Geometry: final body of the model. Coordinates: model frame, mm. A direction names the side the tool comes from. Give positions to 0.01 mm unless a question says otherwise; leave off trailing zeros. Write each loop counter-clockwise with the first axis right and the second up, starting at its lowest first coordinate (ties: lowest second). Pieces come first, ordered by that corner, then holes.
Q1. Section A-A (x = 4). Return the cut outline in (y, z), plus the area to 3 significant figures.
Q2. Section D-D (z = 18). Return the cut outline in (x, y).
Q3. Pin query (flat end, axial travel): pin 1 Ø7 at (y, z) = (-32.5, 15.5) entering from -X; pin 2 Ø9.5 at (y, z) = (-31, -15.5) entering from -X; pin 3 Ø12 at (y, z) = (-10.5, -20) entering from -X. Return the tip coordinate at first contact, or that it passes through.
Q4. Reachability of faces 1 (the flat face through (7.5, -28, -17)), 2 (the flat face through (0, 28, -12.5)), 3 (the flat face through (7.5, 28, 17)), 4 (the cylindrical face through (22.497, -27.325, -0.388)), 5 (the cylindrical face through (-22.497, -27.325, 0.388)) from +Z, -Z, +X, -X, +Y, -Y: full face, straight path, thin tool, end or side. Return the list, or none.
Q5. Mould query, pull axis X, two halves, no side actions, for faces 6 (the flat face through (0, -28, 12.5)), 7 (the flat face through (0, -28, -12.5)), 8 (the cylindrical face through (30, 0, 0)), 9 (the cylindrical face through (-30, 0, 0)). Classes: +X half, -X half, draft (parallel to the pull), parting line (faces both ways), or undercut.
Q6. Section C-C (z = -14.5). Return the cut outline in (x, y), plus the area to 3 significant figures.
Q7. Line query: line 1 (X direction, y = -24, z = 7.5); line 2 (Y direction, x = 8.5, z = -23.5); line 3 (Z direction, x = 7, y = -20). Output: solid intervals per line, ascending.
Q8. Section B-B (y = -20). Return the cut outline in (x, z), plus the area to 3 significant figures.
from build123d import *

# Parameters (mm, degrees)
F0_R     = 30
F1_DEPTH = 15
F2_R     = 22.5
F3_DEPTH = 25
F4_R     = 22.5
F5_DEPTH = 25
F6_W     = 30
F6_H     = 8
F7_DEPTH = 15
F8_W     = 15
F8_H     = 12
F9_DEPTH = 25


# Not quite as in the source:
# - a pattern or mirror of a feature is missing from the dataset's text; its kind, count and spacing are read off the source's solid


with BuildPart() as f1:
    # F0 (on Front) → F1 (new body, symmetric)
    with BuildSketch(Plane.XZ):
        Circle(F0_R)
    extrude(amount=F1_DEPTH, both=True)

    # F2 (on face) → F3 (join)
    with BuildSketch(Plane.XZ.offset(15)):
        Circle(F2_R)
    extrude(amount=F3_DEPTH)

    # F4 (on face) → F5 (join)
    with BuildSketch(Plane(origin=(0, 15, 0), x_dir=(-1, 0, 0), z_dir=(0, 1, 0))):
        Circle(F4_R)
    extrude(amount=F5_DEPTH)

    # F6 (on Front) → F7 (cut, symmetric)
    with BuildSketch(Plane.XZ):
        with Locations((0, 31.5)):
            Rectangle(F6_W, F6_H)
        with Locations((0, -31.5)):
            Rectangle(F6_W, F6_H)
    extrude(amount=F7_DEPTH, both=True, mode=Mode.SUBTRACT)

    # F8 (on face) → F9 (cut)
    with BuildSketch(Plane.XZ.offset(40)):
        with Locations((0, 18.5)):
            Rectangle(F8_W, F8_H)
        with Locations((0, -18.5)):
            Rectangle(F8_W, F8_H)
    f9 = extrude(amount=-F9_DEPTH, mode=Mode.SUBTRACT)

    # F9_copies: F9 across plane
    add(f9.mirror(Plane.ZX), mode=Mode.SUBTRACT)


solid = f1.part
Computed:
1. outline: (-40, -12.5) - (-15, -12.5) - (-15, -27.5) - (15, -27.5) - (15, -12.5) - (40, -12.5) - (40, 12.5) - (15, 12.5) - (15, 27.5) - (-15, 27.5) - (-15, 12.5) - (-40, 12.5) - close
1. area: 2,900 mm2
2. outline: (-24, -15) - (-13.5, -15) - (-13.5, -40) - (-7.5, -40) - (-7.5, -15) - (7.5, -15) - (7.5, -40) - (13.5, -40) - (13.5, -15) - (24, -15) - (24, 15) - (13.5, 15) - (13.5, 40) - (7.5, 40) - (7.5, 15) - (-7.5, 15) - (-7.5, 40) - (-13.5, 40) - (-13.5, 15) - (-24, 15) - close
3. pin 1: stops at x = -19.03
3. pin 2: stops at x = -19.77
3. pin 3: stops at x = -26.53
4. face 1: -Z, -Y
4. face 2: -Z, +Y
4. face 3: +Z, +Y
4. face 4: +X, -Y
4. face 5: -X, -Y
5. face 6: undercut
5. face 7: undercut
5. face 8: +X half
5. face 9: -X half
6. outline: (-26.26, -15) - (-17.2, -15) - (-17.2, -40) - (-7.5, -40) - (-7.5, -15) - (7.5, -15) - (7.5, -40) - (17.2, -40) - (17.2, -15) - (26.26, -15) - (26.26, 15) - (17.2, 15) - (17.2, 40) - (7.5, 40) - (7.5, 15) - (-7.5, 15) - (-7.5, 40) - (-17.2, 40) - (-17.2, 15) - (-26.26, 15) - close
6. area: 2,550 mm2
7. line 1: x = -21.21 to 21.21
7. line 2: y = -15 to 15
7. line 3: z = -12.5 to 12.5
8. outline: (-7.5, -21.21) - (-7.5, -12.5) - (7.5, -12.5) - (7.5, -21.21) arc R22.5 ccw to (7.5, 21.21) - (7.5, 12.5) - (-7.5, 12.5) - (-7.5, 21.21) arc R22.5 ccw to start
8. area: 1,300 mm2
